CAD build for the part. Positions are in the model's coordinates, mm. Round coordinates to 2 decimals unless told otherwise and drop trailing zeros. Order: outer loops, then holes, each group sorted by start corner. A loop starts at its lowest first (then second) coordinate and runs counter-clockwise, first axis right, second up. Notation, with made-up numbers: (72.5, -39) - (124.5, -39) arc R19 ccw to (124.5, -10) - close; hole circle Ø7 at (-12.5, -25). An arc over 180 degrees is marked (long way). Write item = value, one per line.
from build123d import *

# Parameters (mm, degrees)
BOSS_EXTRUDE1_DEPTH = 75


with BuildPart() as part:
    # Sketch1 → Boss-Extrude1 (new body)
    with BuildSketch(Plane(origin=(0, 0, 0), x_dir=(0, 0, -1), z_dir=(1, 0, 0))):
        with BuildLine():
            ThreePointArc((200, 0), (141.421356237, 141.421356237), (0, 200))
            Line((0, 200), (0, 198.4))
            ThreePointArc((0, 198.4), (140.289985387, 140.289985387), (198.4, 0))
            ThreePointArc((198.4, 0), (140.289985387, -140.289985387), (0, -198.4))
            Line((0, -198.4), (0, -200))
            ThreePointArc((0, -200), (141.421356237, -141.421356237), (200, 0))
        make_face()
    extrude(amount=BOSS_EXTRUDE1_DEPTH)


solid = part.part
(1) Band-saw the part on C-C on z = -184. List the corners of the cut face in (x, y).
Solved:
outline = (0, -78.38) - (75, -78.38) - (75, -74.21) - (0, -74.21) - close; (0, 74.21) - (75, 74.21) - (75, 78.38) - (0, 78.38) - close
(2) Drop flat-ended pins along their axis: pin 1 (8 mm diameter, centred on x = 39, y = -88.5, fed in from -Z); pin 2 (5 mm diameter, centred on x = 64.5, z = -108, fed in from +Y); pin 3 (5 mm diameter, centred on x = 41.5, y = 67, fed in from +Z). Give the stop position or say it passes through.
Solved:
pin_1 = -181.27
pin_2 = 169.91
pin_3 = -185.83
(3) Band-saw the part on D-D on y = 101. List the corners of the cut face in (x, z), plus the area to 3 significant figures.
Solved:
outline = (0, -172.62) - (75, -172.62) - (75, -170.77) - (0, -170.77) - close
area = 139 mm²
(4) Probe line 1 along Y through (x, z) = (65.5, -82); line 2 along Y through (x, z) = (26, -61); line 3 along Z through (x, y) = (12.5, -114.5). List the from-to ranges inside material, lowest first.
Solved:
line_1 = -182.42 to -180.66, 180.66 to 182.42
line_2 = -190.47 to -188.79, 188.79 to 190.47
line_3 = -163.98 to -162.03
(5) Band-saw the part on B-B on x = 42. List the corners of the cut face in (y, z), plus the area to 3 significant figures.
Solved:
outline = (-200, 0) arc R200 ccw to (200, 0) - (198.4, 0) arc R198.4 cw to (-198.4, 0) - close
area = 1,000 mm²
(6) Band-saw the part on A-A on z = -73.5. List the corners of the cut face in (x, y), plus the area to 3 significant figures.
Solved:
outline = (0, -186) - (75, -186) - (75, -184.28) - (0, -184.28) - close; (0, 184.28) - (75, 184.28) - (75, 186) - (0, 186) - close
area = 258 mm²
